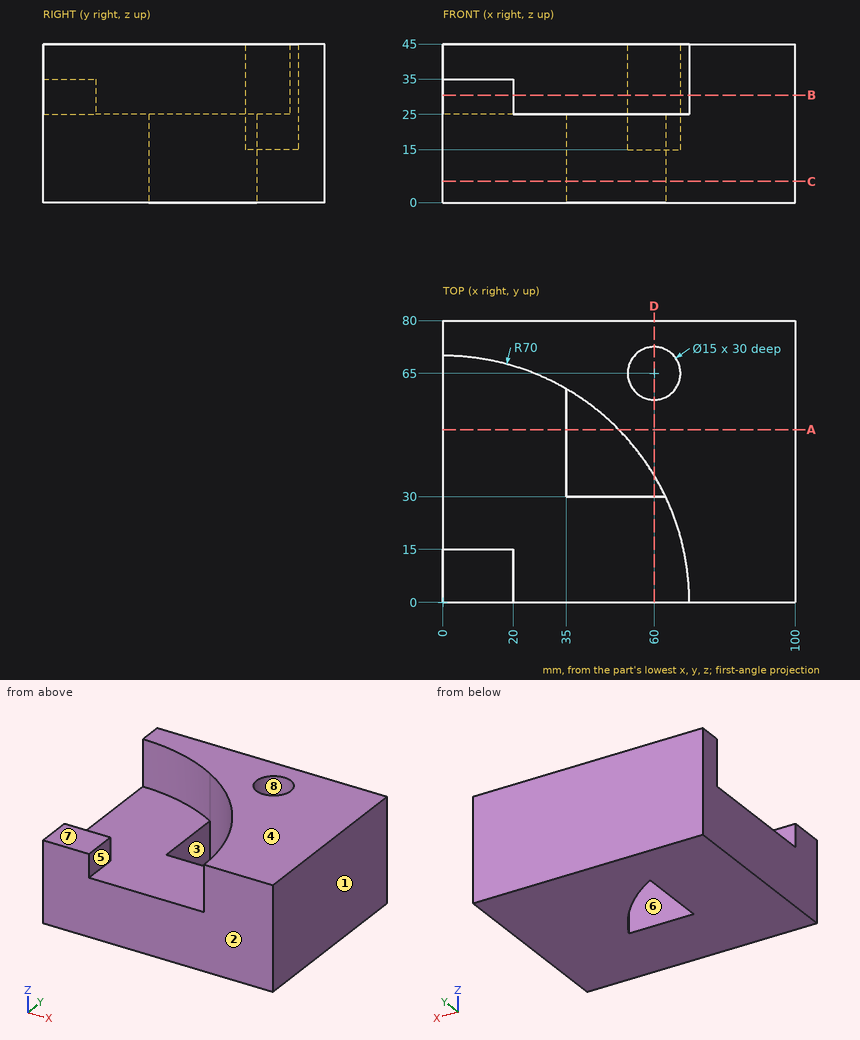
Study the drawing (mm; zero at the part's minimum x, y, z) and answer. A direction names the side the tool comes from. Round coordinates to 2 decimals unless told otherwise and drop trailing zeros. Order: outer loops, then holes, each group sorted by start corner. A loop starts at its lowest first (then second) coordinate and runs counter-clockwise, first axis right, second up. Notation, with made-up numbers: (-35.5, 64.5) -> (6.5, 64.5) arc R27 ccw to (6.5, 85.5) -> close; hole circle Ø9 at (-18.75, -29). An arc over 180 degrees is marked (long way). Answer as CSV lines item,"result". Start each with the question number.
(1) The part is cut by section D-D (x = 60). Determine the outline of the cut face in (y, z).
(2) A tool of negligible diameter and unlimited length cuts with its end or side. For the marked faces 4, 5, 6, 7 and 8, from which of +Z, -Z, +X, -X, +Y, -Y can it reach the whole face along a straight path? Write none if from no direction.
(3) The part is cut by section C-C (z = 6). Determine the outline of the cut face in (x, y), then the cut area to 3 significant figures.
(4) Flat-ended cylindrical pins translate along their axes: pin 1 Ø3 at (y, z) = (41, 36.5) entering from -X; pin 2 Ø21 at (x, y) = (49, 20.5) entering from +Z; pin 3 Ø12 at (x, y) = (13.5, 7) entering from +Z. Find the tip coordinate at first contact, or state that the pin passes through.
(5) The part is cut by section B-B (z = 30.5). Determine the outline of the cut face in (x, y).
(6) Find the intervals of material crossed by probe 1 along Y at (x, z) = (60, 23.5); probe 2 along Z at (x, y) = (65, 22); probe 3 along X at (y, z) = (65, 29), in increasing order. Write a range as from..to.
(7) For a pull along Y with two mould halves and no side action, classify the marked faces 1, 2 and 3 as +Y half, -Y half, draft (parallel to the pull), parting line (faces both ways), or undercut.
(8) The part is cut by section A-A (y = 49). Determine the outline of the cut face in (x, z), then the cut area to 3 significant figures.
Evaluation:
1,outline,"(0, 0) -> (30, 0) -> (30, 25) -> (0, 25) -> close; (36.06, 0) -> (80, 0) -> (80, 45) -> (72.5, 45) -> (72.5, 15) -> (57.5, 15) -> (57.5, 45) -> (36.06, 45) -> close"
2,face 4,"+Z, +X, -X, +Y, -Y"
2,face 5,"+Z, -Y"
2,face 6,"+Z, -Z"
2,face 7,"+Z, -X, -Y"
2,face 8,"+Z"
3,outline,"(0, 0) -> (100, 0) -> (100, 80) -> (0, 80) -> close; hole (35, 30) -> (63.25, 30) arc R70 ccw to (35, 60.62) -> close"
3,area,"7,480 mm²"
4,pin 1,"x = 55.62"
4,pin 2,"z = 25"
4,pin 3,"z = 35"
5,outline,"(0, 0) -> (20, 0) -> (20, 15) -> (0, 15) -> close; (0, 70) arc R70 cw to (70, 0) -> (100, 0) -> (100, 80) -> (0, 80) -> close; hole circle Ø15 at (60, 65)"
6,probe 1,"0..30, 36.06..57.5, 72.5..80"
6,probe 2,"0..25"
6,probe 3,"25.98..52.5, 67.5..100"
7,face 1,"draft"
7,face 2,"-Y half"
7,face 3,"undercut"
8,outline,"(0, 0) -> (35, 0) -> (35, 25) -> (0, 25) -> close; (49.99, 0) -> (100, 0) -> (100, 45) -> (49.99, 45) -> close"
8,area,"3,130 mm²"
